Verification items for the finished model (mm, model axes). Face numbers are marked on the shaded views. A direction names the side the tool comes from. Give positions to 0.01 mm unless a question says otherwise; leave off trailing zeros. Order: outer loops, then holes, each group sorted by start corner. A loop starts at its lowest first (then second) coordinate and runs counter-clockwise, first axis right, second up.
(1) Access from +Z, -Z, +X, -X, +Y, -Y to the whole of each face (thin tool, end or side, straight path). Record for the marked faces 1, 2, 3, 4 and 5.
(2) Sectioned sample at B-B on z = -1.6. Record the cut outline in (x, y), plus the area to 3 significant figures.
(3) Gauge pin test, flat ends, axial feed: pin 1 (0.8 mm diameter, centred on x = -13.5, z = -3.5, fed in from -Y); pin 2 (0.6 mm diameter, centred on x = 10, y = 1, fed in from -Z). Record the tip position at first contact, or that the pin passes through.
(4) Mould release check, pull along X, two halves, no side actions. Record for the marked faces 6, 7, 8 and 9: pulls with the +X half, pulls with the -X half, needs draft (parallel to the pull), parting line crosses it, or undercut.
(5) Sectioned sample at D-D on x = 11.75. Record the cut outline in (y, z), plus the area to 3 significant figures.
(6) Sectioned sample at A-A on y = -0.85. Record the cut outline in (x, z), plus the area to 3 significant figures.
(7) Scan lines: L1, parallel to X at y = 1.5, z = -2.85; L2, parallel to X at y = 1.7, z = -2.65; L3, parallel to X at y = -1.2, z = -0.8. Record each from-to range of solid material in increasing order.
(8) Sectioned sample at C-C on x = 1.75. Record the cut outline in (y, z), plus the area to 3 significant figures.
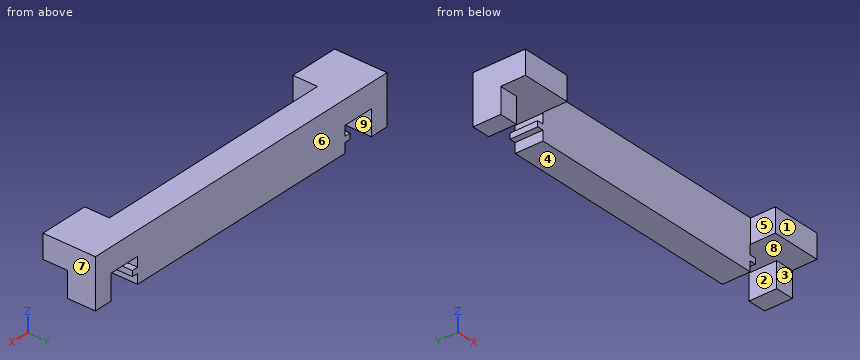
```python
from build123d import *

# Parameters (mm, degrees)
Y_KSEKLIK_EKSTR_ZYON1_DEPTH = 2.25
IZIM5_W                     = 4
IZIM5_H                     = 1.92
Y_KSEKLIK_EKSTR_ZYON4_DEPTH = 2


with BuildPart() as part:
    # Çizim1 → Yükseklik-Ekstrüzyon1 (new body)
    with BuildSketch(Plane(origin=(0, 0, 0), x_dir=(1, 0, 0), z_dir=(0, 1, 0))):
        Polygon((-14, 3.985440092), (-14, 0.015440092), (14, 0.015440092), (14, 3.985440092), (12.5, 3.985440092), (12.5, 1.935440092), (9.95, 1.935440092), (9.95, 2.735440092), (10.45, 2.735440092), (10.45, 3.185440092), (9.95, 3.185440092), (9.95, 3.985440092), (-9.95, 3.985440092), (-9.95, 3.185440092), (-10.45, 3.185440092), (-10.45, 2.735440092), (-9.95, 2.735440092), (-9.95, 1.935440092), (-12.5, 1.935440092), (-12.5, 3.985440092), align=None)
    extrude(amount=Y_KSEKLIK_EKSTR_ZYON1_DEPTH)

    # Çizim5 → Yükseklik-Ekstrüzyon4 (add)
    with BuildSketch(Plane.XZ):
        with Locations((-12, -0.975440092)):
            Rectangle(IZIM5_W, IZIM5_H)
        with Locations((12, -0.975440092)):
            Rectangle(IZIM5_W, IZIM5_H)
    extrude(amount=Y_KSEKLIK_EKSTR_ZYON4_DEPTH)


solid = part.part
```
Ans:
1. face 1: +Z, -Z, +X, -X, -Y
1. face 2: -Z, +Y, -Y
1. face 3: -Z, +X, -X, -Y
1. face 4: -Z, +X, -X, +Y, -Y
1. face 5: +Z, -Z, -Y
2. outline: (-14, -2) - (-10, -2) - (-10, 0) - (10, 0) - (10, -2) - (14, -2) - (14, 2.25) - (-14, 2.25) - close
2. area: 79.0 mm2
3. pin 1: stops at y = 0
3. pin 2: stops at z = -3.99
4. face 6: needs draft
4. face 7: pulls with the +X half
4. face 8: undercut
4. face 9: undercut
5. outline: (-2, -1.94) - (2.25, -1.94) - (2.25, -0.02) - (-2, -0.02) - close
5. area: 8.16 mm2
6. outline: (-14, -1.94) - (-10, -1.94) - (-10, -0.02) - (-14, -0.02) - close; (10, -1.94) - (14, -1.94) - (14, -0.02) - (10, -0.02) - close
6. area: 15.4 mm2
7. L1: x = -14 to -12.5, -10.45 to 10.45, 12.5 to 14
7. L2: x = -14 to -12.5, -9.95 to 9.95, 12.5 to 14
7. L3: x = -14 to -10, 10 to 14
8. outline: (0, -3.99) - (2.25, -3.99) - (2.25, -0.02) - (0, -0.02) - close
8. area: 8.93 mm2
